Source: CAD feature listing. Evaluate the final solid. Frame: model axes, mm. Round coordinates to 2 decimals unless told otherwise and drop trailing zeros. Write each loop counter-clockwise with the first axis right and the second up, starting at its lowest first coordinate (ties: lowest second). Pieces come first, ordered by that corner, then holes. Notation, with made-up numbers: (82.25, -26.5) - (93.25, -26.5) arc R5 cw to (93.25, -18.5) - close; hole circle Ø10 at (33.5, -36). An arc over 180 degrees is marked (long way). Write item = value, one per line. Start each with the question number.
```python
from build123d import *

# Parameters (mm, degrees)
SKETCH1_R           = 0.5
BOSS_EXTRUDE2_DEPTH = 15.5
SKETCH1_3_R         = 1.2
SKETCH1_3_R_2       = 0.5
BOSS_EXTRUDE3_DEPTH = 4.75
FILLET1_R           = 0.2
SKETCH2_R           = 0.85
BOSS_EXTRUDE4_DEPTH = 0.3
SKETCH4_W           = 0.452177067
SKETCH4_H           = 0.051188015
SKETCH5_W           = 2.336260119
SKETCH5_H           = 2.46


with BuildPart() as part:
    # Sketch1 → Boss-Extrude2 (new body)
    with BuildSketch(Plane.XY):
        Circle(SKETCH1_R)
    extrude(amount=BOSS_EXTRUDE2_DEPTH)



with BuildPart() as body_2:
    # Sketch1_3 → Boss-Extrude3 (new body)
    # profile 1 of 2: a face of its own
    with BuildSketch(Plane.XY):
        Circle(SKETCH1_3_R)
        Circle(SKETCH1_3_R_2, mode=Mode.SUBTRACT)
    # profile 2 of 2: a face of its own
    with BuildSketch(Plane.XY):
        Circle(SKETCH1_3_R_2)
    extrude(amount=-BOSS_EXTRUDE3_DEPTH)

    # Fillet1
    fillet1_edges = [body_2.edges().sort_by_distance(p)[0] for p in [
        (-1.2, 0, 0),
    ]]
    fillet(fillet1_edges, radius=FILLET1_R)


with BuildPart() as part_1:
    add(part.part)

    add(body_2.part)  # Boss-Extrude4 merges body 2
    # Sketch2 → Boss-Extrude4 (add)
    with BuildSketch(Plane.XY):
        Circle(SKETCH2_R)
    extrude(amount=BOSS_EXTRUDE4_DEPTH)

    # Sketch3 → Revolve1 (revolve)
    with BuildSketch(Plane(origin=(0, 0, 0), x_dir=(1, 0, 0), z_dir=(0, 1, 0)), mode=Mode.PRIVATE) as revolve1_sk:
        with BuildLine():
            Line((0.5, -15.5), (0, -15.5))
            Line((0, -15.5), (0, -16.0775))
            ThreePointArc((0, -16.0775), (0.247487373, -16.180012627), (0.35, -16.4275))
            Line((0.35, -16.4275), (0.5, -16.4275))
            ThreePointArc((0.5, -16.4275), (0.485692665, -16.308745486), (0.443589461, -16.196787213))
            Line((0.443589461, -16.196787213), (0.443589461, -16.0775))
            Line((0.443589461, -16.0775), (0.535097449, -16.0775))
            Line((0.535097449, -16.0775), (0.535097449, -15.770986484))
            Line((0.535097449, -15.770986484), (0.388145342, -15.770986484))
            ThreePointArc((0.388145342, -15.770986484), (0.417208297, -15.624404477), (0.5, -15.5))
        make_face()
    revolve(revolve1_sk.sketch.rotate(Axis((0, 0, 15.5), (0, 0, 1)), 180), axis=Axis((0, 0, 15.5), (0, 0, 1)))

    # Sketch4 → Revolve2 (revolve)
    with BuildSketch(Plane(origin=(0, 0, 0), x_dir=(1, 0, 0), z_dir=(0, 1, 0))):
        with Locations((-0.226088534, -16.314405992)):
            Rectangle(SKETCH4_W, SKETCH4_H)
    revolve(axis=Axis((0, 0, 16.34), (0, 0, -1)))

    # Sketch5 → Cut-Revolve1 (revolve, cut)
    with BuildSketch(Plane(origin=(0, 0, 0), x_dir=(1, 0, 0), z_dir=(0, 1, 0))):
        with Locations((-1.31613006, -14.27)):
            Rectangle(SKETCH5_W, SKETCH5_H)
    revolve(axis=Axis((0, 0, 16.4275), (0, 0, -1)), mode=Mode.SUBTRACT)


solid = part_1.part
```
(1) Contact query for a flat-ended pin moving along its axis: P1, Ø0.9, axis at x = 0, y = 0, coming from the +Z side. Output: stop coordinate, or through.
(2) Ray query, L1, parallel to Y at x = -0.05, z = 5.5; L2, parallel to Z at x = 0.4, y = 0.85. Return the intervals inside material, ascending. Write a range as from..to.
(3) Pull-direction query (Z, two-part tool) for faces 1 (the cylindrical face through (0.65, 1.01, -2.44)), 2 (the cylindrical face through (-0.108, -0.488, 6.581)), 3 (the flat face through (0, 0, -4.75)); classes: +Z half, -Z half, draft (parallel to the pull), parting line (faces both ways), or undercut.
(4) Section A-A (z = 13.75). Return the cut outline in (x, y), plus the area to 3 significant figures.
Solution:
q1.P1 = 16.43
q2.L1 = -0.5..0.5
q2.L2 = -4.75..0
q3.face_1 = draft
q3.face_2 = undercut
q3.face_3 = -Z half
q4.outline = circle Ø0.3 at (0, 0)
q4.area = 0.0688 mm^2
